Can you work these out from the model? Positions are in its coordinate system, mm. A direction names the side the tool comes from. Coordinates: 2 decimals unless noted, no trailing zeros. Write each loop counter-clockwise with the first axis right and the second up, starting at its lowest first coordinate (ties: lowest second). Pieces come first, ordered by that corner, then holes. Notation, with made-up numbers: (79.5, -29) - (97.5, -29) arc R9 ccw to (97.5, -19) - close; hole circle Ø4 at (18.5, -20.5). An arc over 180 degrees is marked (long way). One line per question, with ' | ' between items. Start each with the question number.
Autodesk Inventor part; units mm, degrees
ref_plane "YZ Plane" through (0, 0, 0) normal (1, 0, 0) x (0, 1, 0)
ref_plane "XZ Plane" through (0, 0, 0) normal (0, 1, 0) x (-1, 0, 0)
ref_plane "XY Plane" through (0, 0, 0) normal (0, 0, 1) x (1, 0, 0)
sketch "Sketch1" plane through (0, 0, 0) normal (0, 0, 1) x (1, 0, 0)
  line L0 (349.5941, 169.6239) -> (430.3941, 169.6239)
  line L1 (430.3941, 209.6239) -> (349.5941, 209.6239)
  line L2 (349.5941, 209.6239) -> (349.5941, 212.7989)
  line L3 (349.5941, 212.7989) -> (339.5941, 212.7989)
  line L4 (339.5941, 212.7989) -> (339.5941, 212.7989)
  line L5 (430.3941, 209.6239) -> (430.3941, 212.7989)
  line L6 (430.3941, 212.7989) -> (440.3941, 212.7989)
  line L7 (440.3941, 212.7989) -> (440.3941, 212.7989)
  line L8 (349.5941, 169.6239) -> (349.5941, 166.4489)
  line L9 (349.5941, 166.4489) -> (339.5941, 166.4489)
  line L10 (339.5941, 166.4489) -> (339.5941, 172.7989)
  line L11 (430.3941, 169.6239) -> (430.3941, 166.4489)
  line L12 (430.3941, 166.4489) -> (440.3941, 166.4489)
  line L13 (440.3941, 166.4489) -> (440.3941, 172.7989)
  line L14 (339.5941, 194.6239) -> (345.9441, 194.6239)
  line L15 (345.9441, 194.6239) -> (345.9441, 184.6239)
  line L16 (345.9441, 184.6239) -> (339.5941, 184.6239)
  line L17 (440.3941, 194.6239) -> (434.0441, 194.6239)
  line L18 (434.0441, 194.6239) -> (434.0441, 184.6239)
  line L19 (434.0441, 184.6239) -> (440.3941, 184.6239)
  line L20 (440.3941, 172.7989) -> (440.3941, 184.6239)
  line L21 (440.3941, 194.6239) -> (440.3941, 212.7989)
  line L22 (339.5941, 212.7989) -> (339.5941, 194.6239)
  line L23 (339.5941, 184.6239) -> (339.5941, 172.7989)
  line L24 (389.9941, 209.6239) -> (389.9941, 169.6239)
  point P0 (0, 0)
  point P1 (339.5941, 192.7989)
  point P2 (339.5941, 192.7989)
  point P3 (345.9441, 189.6239)
  point P4 (389.9941, 189.6239)
  point P5 (434.0441, 189.6239)
  dimension "d16" = 6.35
  dimension "d0" = 40
  dimension "d1" = 100.8
  dimension "d2" = 10
  dimension "d3" = 6.35
  dimension "d4" = 6.35
  dimension "d5" = 10
  dimension "d6" = 10
  dimension "d7" = 10
  dimension "d8" = 10
  dimension "d9" = 3.175
  dimension "d10" = 3.175
  dimension "d11" = 3.175
  dimension "d12" = 3.175
  dimension "d13" = 10
  dimension "d14" = 6.35
  dimension "d15" = 6.35
extrude "Extrusion1" add sketch "Sketch1" along normal blind 6.35
properties part number "boxFront"
(1) Which directions (+Z, -Z, +X, -X, +Y, -Y) give clear straight access to the entire face, cutting with the end or side of a thin tool? Please do faces 1 (the face through (389, 190, 6.35)), 2 (the face through (430.394, 211, 3)), 3 (the face through (430.394, 168, 3)), 4 (the face through (343, 194.624, 3)), 5 (the face through (434.044, 190, 3)).
(2) I'm going to push flat-ended pins straight in: pin 1 (3 mm diameter, centred on y = 191, z = 4.5, fed in from +X); pin 2 (1.5 mm diameter, centred on x = 417.5, z = 5.5, fed in from +Y); pin 3 (1.5 mm diameter, centred on x = 370.5, z = 0.5, fed in from -Y). Where does each tip first touch, or does it pass through?
(3) If I drill on probe 1 along Y at (x, z) = (418.5, 0.5); probe 2 along Y at (x, z) = (436.5, 2.75); probe 3 along X at (y, z) = (192, 5.75), over which ranges is the centre line in solid material (lowest first)?
(4) If we section it at C-C on x = 389: List the corners of the cut face in (y, z) for me.
(5) If we section it at A-A on z = 5.25: List the corners of the cut face in (x, y) for me.
(6) If we section it at B-B on y = 190: List the corners of the cut face in (x, z) for me, plus the area to 3 significant figures.
(7) If we mould it in two halves opening along X, with no side actions, what happens to faces 6 (the face through (391, 209.624, 3)), 7 (the face through (435, 166.449, 3)), 8 (the face through (339.594, 204, 3)), 9 (the face through (440.394, 204, 3))? For each: +X half, -X half, draft (parallel to the pull), parting line (faces both ways), or undercut.
Values:
1) face 1: +Z, +X, -X, +Y, -Y | face 2: +Z, -Z, +Y | face 3: +Z, -Z, -Y | face 4: +Z, -Z, -X | face 5: +Z, -Z, +X
2) pin 1: x = 434.04 | pin 2: y = 209.62 | pin 3: y = 169.62
3) probe 1: 169.62 to 209.62 | probe 2: 166.45 to 184.62, 194.62 to 212.8 | probe 3: 345.94 to 434.04
4) outline: (169.62, 0) - (209.62, 0) - (209.62, 6.35) - (169.62, 6.35) - close
5) outline: (339.59, 166.45) - (349.59, 166.45) - (349.59, 169.62) - (430.39, 169.62) - (430.39, 166.45) - (440.39, 166.45) - (440.39, 184.62) - (434.04, 184.62) - (434.04, 194.62) - (440.39, 194.62) - (440.39, 212.8) - (430.39, 212.8) - (430.39, 209.62) - (349.59, 209.62) - (349.59, 212.8) - (339.59, 212.8) - (339.59, 194.62) - (345.94, 194.62) - (345.94, 184.62) - (339.59, 184.62) - close
6) outline: (345.94, 0) - (434.04, 0) - (434.04, 6.35) - (345.94, 6.35) - close | area: 559 mm2
7) face 6: undercut | face 7: draft | face 8: -X half | face 9: +X half
